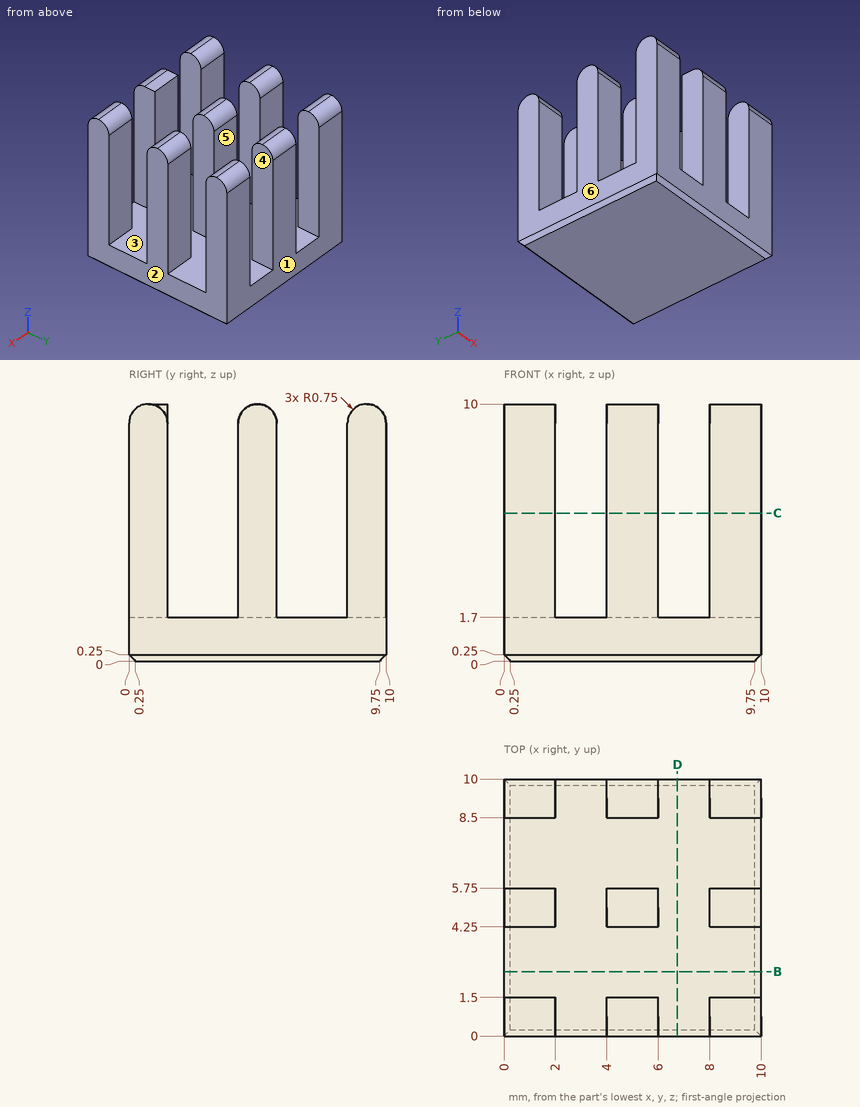
Here's the drawing with two shaded views (mm, measured from the low corner). I have some questions. A direction names the side the tool comes from. Coordinates: 2 decimals unless noted, no trailing zeros. Loops run counter-clockwise (first coordinate to the right, second up) from the corner with the lowest first, then second, coordinate; pieces in that order, holes last. Notation, with made-up numbers: (-34.5, -15.75) -> (19.5, -15.75) arc R10 ccw to (19.5, -2.75) -> close; hole circle Ø2 at (61.5, -9). An arc over 180 degrees is marked (long way). Answer as a JSON object with one key per item and string values.
1) Imagine slicing it at B-B (y = 2.5). Please give me the cut outline in (x, z), then the cut area to 3 significant figures.
Results:
{"outline": "(0, 0.25) -> (0.25, 0) -> (9.75, 0) -> (10, 0.25) -> (10, 1.7) -> (0, 1.7) -> close", "area": "16.9 mm^2"}
2) Thinking about a two-plate mould opening in Y: for the marked faces 1, 2 and 3, which applies, pulls with the +Y half, pulls with the -Y half, needs draft (parallel to the pull), parting line crosses it, or undercut?
Results:
{"face 1": "pulls with the +Y half", "face 2": "needs draft", "face 3": "undercut"}
3) Imagine slicing it at C-C (z = 5.75). Count the separate pieces of the cut face and the enclosed holes in it, then the cut area to 3 significant figures.
Results:
{"separate pieces": "9", "enclosed holes": "0", "area": "27.0 mm^2"}
4) If I drill on line 1 (X direction, y = 0.5, z = 7); line 2 (Y direction, x = 1.5, z = 5.75); line 3 (Z direction, x = 7.5, y = 9), over which ranges is the centre line in solid material (lowest first)?
Results:
{"line 1": "x = 0 to 2, 4 to 6, 8 to 10", "line 2": "y = 0 to 1.5, 4.25 to 5.75, 8.5 to 10", "line 3": "z = 0 to 1.7"}
5) For the marked faces 4, 5 and 6, which set-ups out of +Z, -Z, +X, -X, +Y, -Y let a thin tool reach every point of the face, with its end or its side?
Results:
{"face 4": "+Z, +Y, -Y", "face 5": "+Z, +X, -X", "face 6": "+Z, -Z, -X, +Y, -Y"}
